Geometry: final body of the model. Coordinates: model frame, mm. A direction names the side the tool comes from. Give positions to 0.01 mm unless a question says otherwise; leave off trailing zeros. Write each loop counter-clockwise with the first axis right and the second up, starting at its lowest first coordinate (ties: lowest second). Pieces come first, ordered by that corner, then holes.
from build123d import *

# Parameters (mm, degrees)
F0_R     = 6
F1_DEPTH = 9
F2_R     = 0.5
F3_DEPTH = 7
F4_DEPTH = 5


with BuildPart() as f1:
    # F0 (on Top) → F1 (new body)
    with BuildSketch(Plane.XY):
        Circle(F0_R)
    extrude(amount=F1_DEPTH)

    # F2 (on face) → F3 (join)
    with BuildSketch(Plane(origin=(0, 0, 0), x_dir=(1, 0, 0), z_dir=(0, 0, -1))):
        with Locations((-4.267732, 0)):
            Circle(F2_R)
    extrude(amount=F3_DEPTH)

    # F2 (on face) → F4 (join)
    with BuildSketch(Plane(origin=(0, 0, 0), x_dir=(1, 0, 0), z_dir=(0, 0, -1))):
        with Locations((4.267732, 0)):
            Circle(F2_R)
    extrude(amount=F4_DEPTH)


solid = f1.part
Q1. Section C-C on x = 0. Output: boundary loops of the cut face in (y, z).
Filled sheet:
outline: (-6, 0) - (6, 0) - (6, 9) - (-6, 9) - close
Q2. Pull-direction query (X, two-part tool) for faces 1 (the cylindrical face through (-6, 0, 4)), 2 (the cylindrical face through (4.73, 0.19, -2.46)), 3 (the flat face through (-4, 0, -7)); classes: released by +X, released by -X, zero draft, split by the parting line, or undercut.
Filled sheet:
face 1: split by the parting line
face 2: undercut
face 3: zero draft
Q3. Section A-A on z = -3.25. Output: boundary loops of the cut face in (x, y).
Filled sheet:
outline: circle Ø1 at (-4.27, 0); circle Ø1 at (4.27, 0)
Q4. Ray query, line 1 along X through (y, z) = (0, -4.75); line 2 along Z through (x, y) = (-0.75, 5.25); line 3 along Y through (x, z) = (5.25, 8). Return the intervals inside material, ascending.
Filled sheet:
line 1: x = -4.77 to -3.77, 3.77 to 4.77
line 2: z = 0 to 9
line 3: y = -2.9 to 2.9
Q5. Section B-B on y = 0. Output: boundary loops of the cut face in (x, z), plus the area to 3 significant figures.
Filled sheet:
outline: (-6, 0) - (-4.77, 0) - (-4.77, -7) - (-3.77, -7) - (-3.77, 0) - (3.77, 0) - (3.77, -5) - (4.77, -5) - (4.77, 0) - (6, 0) - (6, 9) - (-6, 9) - close
area: 120 mm2
Q6. Access query for faces 4 (the flat face through (4, 0, -5)), 5 (the cylindrical face through (-3.79, -0.15, -3.45)), 6 (the flat face through (0, 0, 9)). Directions: +Z, -Z, +X, -X, +Y, -Y. A direction counts if a zero-diameter tool reaches every point of the face in a straight line with its end or side. Return the directions, or none.
Filled sheet:
face 4: -Z, +X, +Y, -Y
face 5: -Z
face 6: +Z, +X, -X, +Y, -Y
Q7. Pin query (flat end, axial travel): P1, Ø4, axis at x = 4, y = 2, coming from the -Z side; P2, Ø1, axis at y = -1, z = 0.5, coming from the +X side; P3, Ø3, axis at x = 2.5, z = -4.5, coming from the +Y side. Return the tip coordinate at first contact, or that it passes through.
Filled sheet:
P1: stops at z = -5
P2: stops at x = 5.98
P3: stops at y = 0.42
Q8. Section D-D on z = 6.25. Output: boundary loops of the cut face in (x, y), plus the area to 3 significant figures.
Filled sheet:
outline: circle Ø12 at (0, 0)
area: 113 mm2
